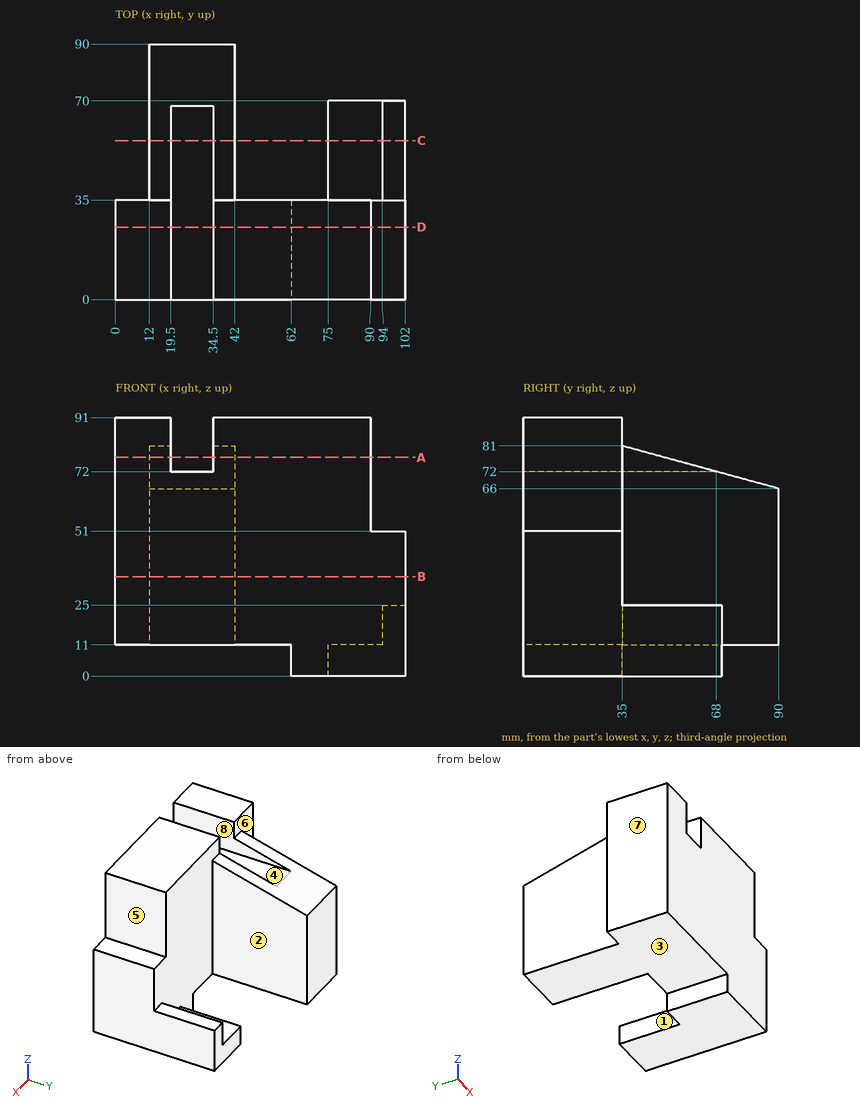
Geometry check sheet. Reference: drawing and pictorial views, mm from the part's lowest x, y, z. A direction names the side the tool comes from. Round coordinates to 2 decimals unless told otherwise and drop trailing zeros. Loops run counter-clockwise (first coordinate to the right, second up) from the corner with the lowest first, then second, coordinate; pieces in that order, holes last. Notation, with made-up numbers: (85, 61) - (91, 61) arc R10 ccw to (91, 71) - close; hole circle Ø10 at (33.5, 51.5). An arc over 180 degrees is marked (long way). Answer as CSV lines item,"result".
(1) Cross-section at D-D, the plane y = 25.5. Enter the section's corners in (x, z), and give its area (4 significant figures).
Output values:
outline,"(0, 11) - (62, 11) - (62, 0) - (102, 0) - (102, 51) - (90, 51) - (90, 91) - (34.5, 91) - (34.5, 72) - (19.5, 72) - (19.5, 91) - (0, 91) - close"
area,"7,835 mm²"
(2) Cross-section at C-C, the plane y = 56. Enter the section's corners in (x, z).
Output values:
outline,"(12, 11) - (42, 11) - (42, 75.27) - (34.5, 75.27) - (34.5, 72) - (19.5, 72) - (19.5, 75.27) - (12, 75.27) - close; (75, 0) - (102, 0) - (102, 25) - (94, 25) - (94, 11) - (75, 11) - close"
(3) Release check for a two-part mould opening along X. For the marked faces 6, 7 and 8 record: released by +X, released by -X, zero draft, split by the parting line, or undercut.
Output values:
face 6,"zero draft"
face 7,"released by -X"
face 8,"undercut"
(4) Cross-section at A-A, the plane z = 77. Enter the section's corners in (x, y), and give its area (4 significant figures).
Output values:
outline,"(0, 0) - (19.5, 0) - (19.5, 49.67) - (12, 49.67) - (12, 35) - (0, 35) - close; (34.5, 0) - (90, 0) - (90, 35) - (42, 35) - (42, 49.67) - (34.5, 49.67) - close"
area,"2,845 mm²"
(5) Set-up check for the marked faces 1, 2, 3, 4 and 5: record each of +Z, -Z, +X, -X, +Y, -Y from which the full face is reachable in a straight line by a thin tool's end or side.
Output values:
face 1,"+Z, -Z, -X, +Y"
face 2,"+Z, -Z, +Y"
face 3,"-Z, -X, +Y, -Y"
face 4,"+Z, +Y, -Y"
face 5,"+Z, +X, +Y, -Y"
(6) Depth check by flat-ended pin: pin 1 Ø4.5 at (x, y) = (25, 43) entering from +Z; pin 2 Ø9 at (y, z) = (21.5, 4) entering from -X; pin 3 Ø9.5 at (y, z) = (36, 84) entering from +X. Enter the tip coordinate at first touch or a pass-through.
Output values:
pin 1,"stops at z = 72"
pin 2,"stops at x = 62"
pin 3,"stops at x = 90"
(7) Material ranges on line 1 along X through (y, z) = (65, 16.5); line 2 along X through (y, z) = (25.5, 78.5); line 3 along Y through (x, z) = (43.5, 67), recorded low to high.
Output values:
line 1,"x = 12 to 42, 94 to 102"
line 2,"x = 0 to 19.5, 34.5 to 90"
line 3,"y = 0 to 35"
(8) Cross-section at B-B, the plane z = 35. Enter the section's corners in (x, y), and give its area (3 significant figures).
Output values:
outline,"(0, 0) - (102, 0) - (102, 35) - (42, 35) - (42, 90) - (12, 90) - (12, 35) - (0, 35) - close"
area,"5,220 mm²"
